Verification items for the finished model (mm, model axes). Round coordinates to 2 decimals unless told otherwise and drop trailing zeros. Order: outer loops, then holes, each group sorted by start corner. A loop starts at its lowest first (then second) coordinate and runs counter-clockwise, first axis right, second up. Notation, with made-up numbers: M 17,61 L 71,61 A21 cw 71,76 Z; hole C 0.25,39 d1. An arc over 180 degrees is marked long. Use one line per item in the form item = value. Start each with the question number.
Item 1: Cross-section at B-B on z = -22.5. Enter the section's corners in (x, y).
Item 2: Thickness scan on probe 1 along X at (y, z) = (0.75, -22.5); probe 2 along Z at (x, y) = (22.5, 0.8); probe 3 along X at (y, z) = (0.55, -2). Record the ranges inside material, lowest first. Write a range as [from, to].
Item 3: Cross-section at A-A on x = 22.5. Enter the section's corners in (y, z).
Item 4: Release check for a two-part mould opening along X. For faces 1 (the cylindrical face through (24.699, 0.811, -0.285)), 2 (the flat face through (13, 1.6, -12)), 3 (the cylindrical face through (1.013, 0.811, -2.305)), 4 (the cylindrical face through (0.285, 0.811, -0.301)) record: +X half, -X half, draft (parallel to the pull), parting line (faces both ways), or undercut.
Item 5: Go/stop test with flat-tipped pins: pin 1 Ø4 at (x, z) = (2.5, -2.5) entering from -Y; pin 2 Ø2.5 at (x, z) = (2.5, -22.5) entering from -Y. Record where each tip stops, or that it passes through.
Item 6: Cross-section at C-C on y = 1.1. Enter the section's corners in (x, z).
Autodesk Inventor part; units mm, degrees
ref_plane "YZ Plane" through (0, 0, 0) normal (1, 0, 0) x (0, 1, 0)
ref_plane "XZ Plane" through (0, 0, 0) normal (0, 1, 0) x (-1, 0, 0)
ref_plane "XY Plane" through (0, 0, 0) normal (0, 0, 1) x (1, 0, 0)
sketch "Sketch1" plane through (0, 0, 0) normal (0, 1, 0) x (-1, 0, 0)
  line L0 (0, 0) -> (-25, 0)
  line L1 (-25, 0) -> (-25, -25)
  line L2 (-25, -25) -> (0, -25)
  line L3 (0, -25) -> (0, 0)
  line L4 (-2.5, -22.5) -> (-22.5, -22.5) construction
  line L5 (-22.5, -22.5) -> (-22.5, -2.5) construction
  line L6 (-22.5, -2.5) -> (-2.5, -2.5) construction
  line L7 (-2.5, -2.5) -> (-2.5, -22.5) construction
  dimension "d0" = 25
  dimension "d1" = 25
  dimension "d2" = 20
  dimension "d3" = 20
  dimension "d4" = 2.5
  dimension "d5" = 2.5
extrude "Extrusion1" add sketch "Sketch1" along normal blind 1.6
hole "Hole1" at (2.5, 0, -22.5) at (2.5, 0, -2.5) at (22.5, 0, -2.5) at (22.5, 0, -22.5) direction (0, 1, 0) diameter 3 depth 8 tip angle 118
fillet "Fillet1" radius 1 4 edges at (25, 0.8, -25) (25, 0.8, 0) (0, 0.8, -25) (0, 0.8, 0)
properties part number "Large Encoder PCB"
Output values:
q1.outline = M 0,0 L 1,0 L 1,1.6 L 0,1.6 Z; M 4,0 L 21,0 L 21,1.6 L 4,1.6 Z; M 24,0 L 25,0 L 25,1.6 L 24,1.6 Z
q2.probe_1 = [0, 1], [4, 21], [24, 25]
q2.probe_2 = [-25, -24], [-21, -4], [-1, 0]
q2.probe_3 = [0, 1.09], [3.91, 21.09], [23.91, 25]
q3.outline = M 0,-25 L 1.6,-25 L 1.6,-24 L 0,-24 Z; M 0,-21 L 1.6,-21 L 1.6,-4 L 0,-4 Z; M 0,-1 L 1.6,-1 L 1.6,0 L 0,0 Z
q4.face_1 = +X half
q4.face_2 = draft
q4.face_3 = undercut
q4.face_4 = -X half
q5.pin_1 = 0
q5.pin_2 = through
q6.outline = M 0,-24 A1 ccw 1,-25 L 24,-25 A1 ccw 25,-24 L 25,-1 A1 ccw 24,0 L 1,0 A1 ccw 0,-1 Z; hole C 2.5,-22.5 d3; hole C 2.5,-2.5 d3; hole C 22.5,-22.5 d3; hole C 22.5,-2.5 d3
